Source: three-view drawing plus pictorial views. Frame: mm from the lowest corner of the part. Round coordinates to 2 decimals unless told otherwise and drop trailing zeros. Loops run counter-clockwise (first coordinate to the right, second up) from the corner with the lowest first, then second, coordinate; pieces in that order, holes last. Notation, with made-up numbers: (-3.75, 17) -> (38.25, 17) arc R20 ccw to (38.25, 56) -> close; hole circle Ø9 at (76.25, 65). An arc over 180 degrees is marked (long way). Put each result on its own line as item: value. Start each with the question number.
1. Material intervals for L1, parallel to Y at x = 11.5, z = 19.5; L2, parallel to X at y = 14.75, z = 17; L3, parallel to Y at x = 13.5, z = 6, sorted ascending.
2. Cut plane C-C (x = 18.5). Return the cut outline in (y, z).
3. Cut plane B-B (y = 7). Return the cut outline in (x, z).
4. Cut plane A-A (z = 11.25). Return the cut outline in (x, y).
5. Contact query for flat-ended pins moving along their axis: pin 1 (1 mm diameter, centred on x = 17, z = 10.5, fed in from +Y); pin 2 (1 mm diameter, centred on y = 13.5, z = 15.5, fed in from -X); pin 3 (12 mm diameter, centred on y = 13, z = 22.5, fed in from -X); pin 4 (1 mm diameter, centred on x = 17, z = 15, fed in from -Y). Output: stop coordinate, or through.
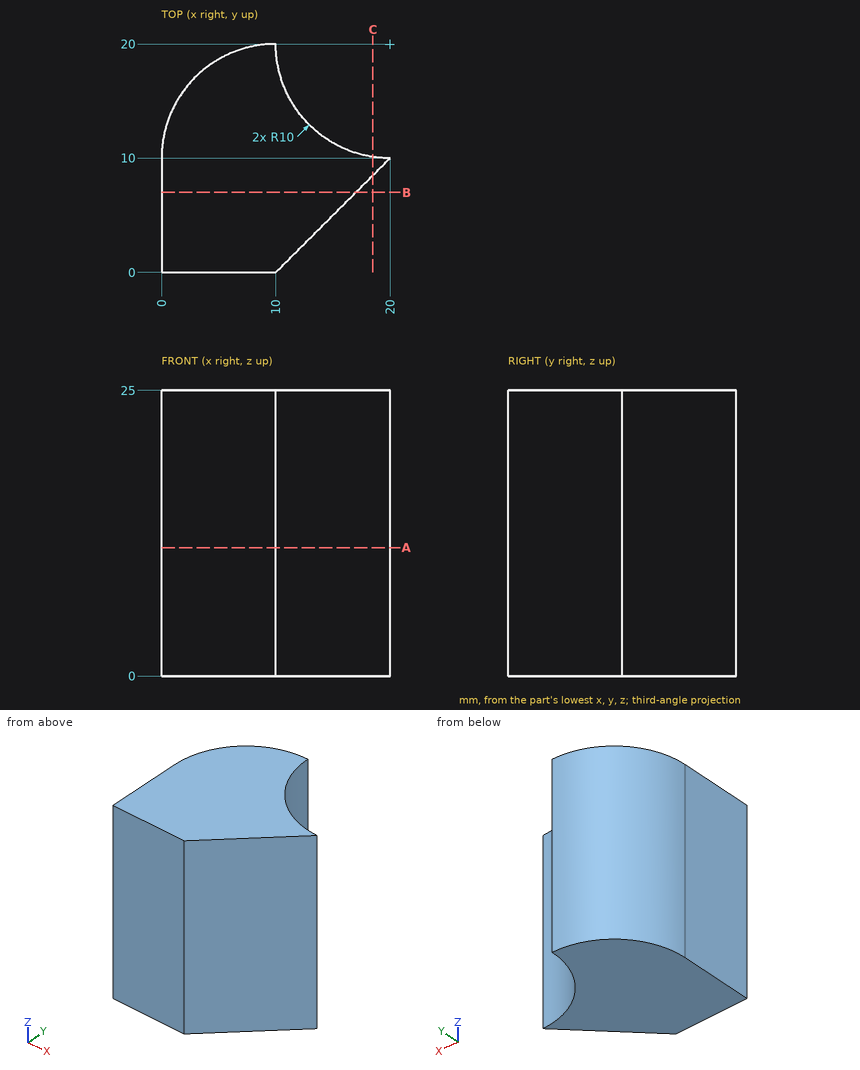
Solution:
1. L1: y = 1.5 to 14.73
1. L2: x = 1.2 to 11.49
1. L3: y = 3.5 to 12.4
2. outline: (8.5, 0) -> (10.11, 0) -> (10.11, 25) -> (8.5, 25) -> close
3. outline: (0, 0) -> (17, 0) -> (17, 25) -> (0, 25) -> close
4. outline: (0, 0) -> (10, 0) -> (20, 10) arc R10 cw to (10, 20) arc R10 ccw to (0, 10) -> close
5. pin 1: stops at y = 10.63
5. pin 2: stops at x = 0.46
5. pin 3: stops at x = 0
5. pin 4: stops at y = 6.5
